```python
from build123d import *

# Parameters (mm, degrees)
BASPROSKE_W         = 15
BASPROSKE_H         = 17
TOOTHCUT_DEPTH      = 29.337254631
TEETHCUTS_COUNT     = 15
TEETHCUTS_ANGLE     = 336
BORSKE_R            = 2.5
BORE_DEPTH          = 50.0000508
SKETCH1_R           = 10
BOSS_EXTRUDE1_DEPTH = 50
CUT_EXTRUDE3_START  = -20
SKETCH2_R           = 2.5
CUT_EXTRUDE3_DEPTH  = 20


with BuildPart() as part:
    # BasProSke → Base-Revolve (revolve)
    with BuildSketch(Plane(origin=(0, 0, 0), x_dir=(1, 0, 0), z_dir=(0, 1, 0)), mode=Mode.PRIVATE) as base_revolve_sk:
        with Locations((7.5, 8.5)):
            Rectangle(BASPROSKE_W, BASPROSKE_H)
    revolve(base_revolve_sk.sketch.rotate(Axis((-10, 0, 0), (1, 0, 0)), 180), axis=Axis((-10, 0, 0), (1, 0, 0)))

    # TooCutSke → ToothCut (cut, through all)
    with BuildSketch(Plane(origin=(0, 0, 0), x_dir=(0, 0, -1), z_dir=(1, 0, 0))):
        with BuildLine():
            ThreePointArc((1.050056448, 12.454813626), (0, 12.499), (-1.050056448, 12.454813626))
            ThreePointArc((-1.050056448, 12.454813626), (-1.638118106, 14.809604533), (-3.110934279, 16.73876737))
            ThreePointArc((-3.110934279, 16.73876737), (0, 17.0254), (3.110934279, 16.73876737))
            ThreePointArc((3.110934279, 16.73876737), (1.638118106, 14.809604533), (1.050056448, 12.454813626))
        make_face()
    toothcut = extrude(amount=TOOTHCUT_DEPTH, mode=Mode.SUBTRACT)

    # TeethCuts: ToothCut ×15 about axis
    teethcuts_axis = Axis((-10, 0, 0), (1, 0, 0))
    for i in range(1, TEETHCUTS_COUNT):
        add(toothcut.rotate(teethcuts_axis, i * TEETHCUTS_ANGLE / (TEETHCUTS_COUNT - 1)), mode=Mode.SUBTRACT)

    # BorSke → Bore (cut, symmetric)
    with BuildSketch(Plane(origin=(0, 0, 0), x_dir=(0, 0, -1), z_dir=(1, 0, 0))):
        with Locations(Location((0, 0, 0), (0, 0, 180))):
            Circle(BORSKE_R)
    extrude(amount=BORE_DEPTH, both=True, mode=Mode.SUBTRACT)

    # Sketch1 → Boss-Extrude1 (add)
    with BuildSketch(Plane(origin=(15, 0, 0), x_dir=(0, 0, -1), z_dir=(1, 0, 0))):
        with Locations(Location((0, 0, 0), (0, 0, 180))):
            Circle(SKETCH1_R)
    extrude(amount=BOSS_EXTRUDE1_DEPTH)

    # Sketch2 → Cut-Extrude3 (cut)
    with BuildSketch(Plane.ZY.offset(CUT_EXTRUDE3_START)):
        Circle(SKETCH2_R)
    extrude(amount=CUT_EXTRUDE3_DEPTH, mode=Mode.SUBTRACT)


solid = part.part
```
Verification items for the finished model (mm, model axes). A direction names the side the tool comes from. Coordinates: 2 decimals unless noted, no trailing zeros. Loops run counter-clockwise (first coordinate to the right, second up) from the corner with the lowest first, then second, coordinate; pieces in that order, holes last. Notation, with made-up numbers: (-17, 45) -> (26, 45) arc R21 ccw to (26, 74) -> close; hole circle Ø11 at (25, 61.25). An arc over 180 degrees is marked (long way). Answer in a Markdown table with one row per item. Add a question column.
1. Access from +Z, -Z, +X, -X, +Y, -Y to the whole of each face (thin tool, end or side, straight path). Record for faces 1 (the face through (7.4, -6.26, -10.82)), 2 (the face through (20, 0, 0)), 3 (the face through (7.4, 12.87, -7.53)), 4 (the face through (7.4, -3.15, 14.51)).
2. Section check B-B, the plane y = 4. Enter the section's corners in (x, z).
3. Depth check by flat-ended pin: P1, Ø3, axis at x = 16, y = -8.5, coming from the +Z side; P2, Ø12, axis at x = 55, y = -10, coming from the +Z side; P3, Ø4, axis at x = 23.5, y = 1.5, coming from the +Z side. Enter the tip coordinate at first touch or a pass-through.
4. Draft check along Y on faces 5 (the face through (15, 1.03, 10.12)), 6 (the face through (7.395, 3.016, -14.609)), 7 (the face through (40, 0, -10)), 8 (the face through (7.395, -14.159, 4.692)). Enter one of: +Y half, -Y half, draft (parallel to the pull), parting line (faces both ways), or undercut.
5. Material ranges on probe 1 along Y at (x, z) = (17, 0); probe 2 along Y at (x, z) = (10, 0); probe 3 along X at (y, z) = (0.5, 1.5), recorded low to high. Write a range as [from, to].
6. Section check C-C, the plane x = 55. Enter the section's corners in (y, z), then the cut area to 3 significant figures.
7. Section check A-A, the plane x = 19. Enter the section's corners in (y, z), then the cut area to 3 significant figures.
Derived:
| question | item | result |
|---|---|---|
| 1 | face 1 | +X, -X |
| 1 | face 2 | -X |
| 1 | face 3 | +X, -X, +Y |
| 1 | face 4 | +Z, +X, -X |
| 2 | outline | (0, -11.84) -> (15, -11.84) -> (15, -9.17) -> (65, -9.17) -> (65, 9.17) -> (15, 9.17) -> (15, 11.84) -> (0, 11.84) -> close |
| 3 | P1 | stops at z = 12.46 |
| 3 | P2 | stops at z = 9.17 |
| 3 | P3 | stops at z = 10 |
| 4 | face 5 | draft |
| 4 | face 6 | undercut |
| 4 | face 7 | parting line |
| 4 | face 8 | -Y half |
| 5 | probe 1 | y = [-10, -2.5], [2.5, 10] |
| 5 | probe 2 | y = [-17, -2.5], [2.5, 12.5] |
| 5 | probe 3 | x = [20, 65] |
| 6 | outline | circle Ø20 at (0, 0) |
| 6 | area | 314 mm² |
| 7 | outline | circle Ø20 at (0, 0); hole circle Ø5 at (0, 0) |
| 7 | area | 295 mm² |
